```python
from build123d import *

# Parameters (mm, degrees)
SKETCH1_W           = 15
SKETCH1_H           = 4
BOSS_EXTRUDE1_DEPTH = 15
SKETCH2_W           = 15
SKETCH2_H           = 5
BOSS_EXTRUDE2_DEPTH = 15
FILLET1_R           = 1
FILLET3_R           = 5
SKETCH3_R           = 5
CUT_EXTRUDE1_DEPTH  = 3.2
SKETCH4_R           = 1.6
CUT_EXTRUDE2_DEPTH  = 26.980762229
FILLET4_R           = 5


with BuildPart() as part:
    # Sketch1 → Boss-Extrude1 (new body)
    with BuildSketch(Plane(origin=(0, 0, 0), x_dir=(1, 0, 0), z_dir=(0, 1, 0))):
        with Locations((7.5, 2)):
            Rectangle(SKETCH1_W, SKETCH1_H)
    extrude(amount=BOSS_EXTRUDE1_DEPTH)

    # Sketch2 → Boss-Extrude2 (add)
    with BuildSketch(Plane.XY):
        with Locations((7.5, 12.5)):
            Rectangle(SKETCH2_W, SKETCH2_H)
    extrude(amount=BOSS_EXTRUDE2_DEPTH)

    # Fillet1
    fillet1_edges = [part.edges().sort_by_distance(p)[0] for p in [
        (7.5, 10, 0),
    ]]
    fillet(fillet1_edges, radius=FILLET1_R)

    # Fillet3
    # the kernel refuses this fillet: 5 mm, written as the material it takes off along each edge
    with BuildSketch(Plane(origin=(5, 15, 10), x_dir=(0, -1, 0), z_dir=(-1, 0, 0))) as fillet3_piece_1_section:
        Polygon((0, 0), (FILLET3_R * 1.02, 0), (FILLET3_R * 1.02, FILLET3_R * 1.02), (0, FILLET3_R * 1.02), align=None)
    fillet3_piece_1 = extrude(amount=FILLET3_R * 1.02, mode=Mode.PRIVATE)
    fillet3_piece_1 = fillet3_piece_1 - Plane(origin=(5, 15, 10), x_dir=(0, 0.7071067811865475, -0.7071067811865475), z_dir=(-1, 0, 0)) * Sphere(FILLET3_R, mode=Mode.PRIVATE)
    add(fillet3_piece_1, mode=Mode.SUBTRACT)
    with BuildSketch(Plane(origin=(10, 15, 10), x_dir=(0, -1, 0), z_dir=(1, 0, 0))) as fillet3_piece_2_section:
        Polygon((0, 0), (FILLET3_R * 1.02, 0), (FILLET3_R * 1.02, -FILLET3_R * 1.02), (0, -FILLET3_R * 1.02), align=None)
    fillet3_piece_2 = extrude(amount=FILLET3_R * 1.02, mode=Mode.PRIVATE)
    fillet3_piece_2 = fillet3_piece_2 - Plane(origin=(10, 15, 10), x_dir=(0, 0.7071067811865475, -0.7071067811865475), z_dir=(1, 0, 0)) * Sphere(FILLET3_R, mode=Mode.PRIVATE)
    add(fillet3_piece_2, mode=Mode.SUBTRACT)
    with BuildSketch(Plane(origin=(0, 10, 1), x_dir=(0, 1, 0), z_dir=(0, 0, 1))) as fillet3_piece_3:
        with BuildLine():
            CenterArc((FILLET3_R, -FILLET3_R), FILLET3_R, 90, 90)
            Line((0, -FILLET3_R), (0, 0))
            Line((0, 0), (FILLET3_R, 0))
        make_face()
    extrude(amount=9, mode=Mode.SUBTRACT)
    with BuildSketch(Plane(origin=(15, 10, 1), x_dir=(0, 1, 0), z_dir=(0, 0, 1))) as fillet3_piece_4:
        with BuildLine():
            CenterArc((FILLET3_R, FILLET3_R), FILLET3_R, 180, 90)
            Line((0, FILLET3_R), (0, 0))
            Line((0, 0), (FILLET3_R, 0))
        make_face()
    extrude(amount=9, mode=Mode.SUBTRACT)
    with BuildSketch(Plane(origin=(10, 10, 15), x_dir=(0, 0, -1), z_dir=(-1, 0, 0))) as fillet3_piece_5:
        with BuildLine():
            CenterArc((FILLET3_R, -FILLET3_R), FILLET3_R, 90, 90)
            Line((0, -FILLET3_R), (0, 0))
            Line((0, 0), (FILLET3_R, 0))
        make_face()
    extrude(amount=5, mode=Mode.SUBTRACT)
    with BuildSketch(Plane(origin=(0, -12.5, 0), x_dir=(1, 0, 0), z_dir=(0, 1, 0))) as fillet3_piece_6:
        with BuildLine():
            CenterArc((FILLET3_R, FILLET3_R), FILLET3_R, 180, 90)
            Line((0, FILLET3_R), (0, 0))
            Line((0, 0), (FILLET3_R, 0))
        make_face()
    extrude(amount=21.5, mode=Mode.SUBTRACT)
    with BuildSketch(Plane(origin=(15, -12.5, 0), x_dir=(-1, 0, 0), z_dir=(0, 1, 0))) as fillet3_piece_7:
        with BuildLine():
            CenterArc((FILLET3_R, -FILLET3_R), FILLET3_R, 90, 90)
            Line((0, -FILLET3_R), (0, 0))
            Line((0, 0), (FILLET3_R, 0))
        make_face()
    extrude(amount=21.5, mode=Mode.SUBTRACT)
    with BuildSketch(Plane(origin=(15, 9, 1), x_dir=(0, 0, -1), z_dir=(0, -1, 0))) as fillet3_piece_8:
        with BuildLine():
            CenterArc((1 + FILLET3_R, -FILLET3_R), FILLET3_R, 90, 90)
            Line((1, -FILLET3_R), (1, 0))
            Line((1, 0), (1 + FILLET3_R, 0))
        make_face()
    revolve(axis=Axis((15, 9, 1), (1, 0, 0)), revolution_arc=90, mode=Mode.SUBTRACT)
    with BuildSketch(Plane(origin=(0, 9, 1), x_dir=(0, 0, -1), z_dir=(0, -1, 0))) as fillet3_piece_9:
        with BuildLine():
            CenterArc((1 + FILLET3_R, FILLET3_R), FILLET3_R, 180, 90)
            Line((1 + FILLET3_R, 0), (1, 0))
            Line((1, 0), (1, FILLET3_R))
        make_face()
    revolve(axis=Axis((0, 9, 1), (1, 0, 0)), revolution_arc=90, mode=Mode.SUBTRACT)

    # Sketch3 → Cut-Extrude1 (cut)
    with BuildSketch(Plane(origin=(0, 15, 0), x_dir=(1, 0, 0), z_dir=(0, 1, 0))):
        with Locations(Location((7.5, -6, 0), (0, 0, 270))):
            Circle(SKETCH3_R)
    extrude(amount=-CUT_EXTRUDE1_DEPTH, mode=Mode.SUBTRACT)

    # Sketch4 → Cut-Extrude2 (cut, through all)
    with BuildSketch(Plane.XY):
        with Locations((7.601020514, 5)):
            Circle(SKETCH4_R)
    extrude(amount=-CUT_EXTRUDE2_DEPTH, mode=Mode.SUBTRACT)

    # Fillet4
    # the kernel refuses this fillet: 5 mm, written as the material it takes off along each edge
    with BuildSketch(Plane(origin=(5, 0, -5), x_dir=(0, 0, 1), z_dir=(1, 0, 0))) as fillet4_piece_1:
        with BuildLine():
            CenterArc((5 - FILLET4_R, -FILLET4_R), FILLET4_R, 0, 90)
            Line((5 - FILLET4_R, 0), (5, 0))
            Line((5, 0), (5, -FILLET4_R))
        make_face()
    revolve(axis=Axis((5, 0, -5), (0, -1, 0)), revolution_arc=221.746220733, mode=Mode.SUBTRACT)
    with BuildSketch(Plane(origin=(10, 0, -5), x_dir=(-0.6658324541231062, 0, -0.7461012954260312), z_dir=(-0.7461012954260312, 0, 0.6658324541231062))) as fillet4_piece_2:
        with BuildLine():
            CenterArc((5 - FILLET4_R, -FILLET4_R), FILLET4_R, 0, 90)
            Line((5 - FILLET4_R, 0), (5, 0))
            Line((5, 0), (5, -FILLET4_R))
        make_face()
    revolve(axis=Axis((10, 0, -5), (0, -1, 0)), revolution_arc=221.746220733, mode=Mode.SUBTRACT)
    with BuildSketch(Plane(origin=(5, 0, 0), x_dir=(0, 1, 0), z_dir=(1, 0, 0))) as fillet4_piece_3:
        with BuildLine():
            CenterArc((FILLET4_R, -FILLET4_R), FILLET4_R, 90, 90)
            Line((0, -FILLET4_R), (0, 0))
            Line((0, 0), (FILLET4_R, 0))
        make_face()
    extrude(amount=5, mode=Mode.SUBTRACT)


solid = part.part
```
Work out the finished part from the listing and answer in its coordinate system (mm). A direction names the side the tool comes from. Give positions to 0.01 mm unless a question says otherwise; leave off trailing zeros. Order: outer loops, then holes, each group sorted by start corner. A loop starts at its lowest first (then second) coordinate and runs counter-clockwise, first axis right, second up. Notation, with made-up numbers: M -5.5,23 L 4.5,23 A11 cw 4.5,30 Z; hole C -30,37.5 d9. An arc over 180 degrees is marked long. Return JSON: item names as keys, results as strings.
1) For a pull along X with two mould halves and no side action, classify faces 5 (the flat face through (8, 11.8, 6)), 6 (the cylindrical face through (7.393, 6.586, -1.972)), 7 (the flat face through (7, 10, 5)), 8 (the flat face through (15, 14, -3)) as +X half, -X half, draft (parallel to the pull), parting line (faces both ways), or undercut.
Resolved:
{"face 5": "undercut", "face 6": "undercut", "face 7": "draft", "face 8": "+X half"}
2) Section B-B, the plane y = 3.75 is taken. Write down the section's boundary in (x, z).
Resolved:
{"outline": "M 0.26,-4 L 6.6,-4 L 6.6,-0.16 L 5,-0.16 A4.84 ccw Z; M 8.6,-4 L 14.74,-4 A4.84 ccw 10,-0.16 L 8.6,-0.16 Z"}
3) Straight lines are drawn through the part: line 1 along Y through (x, z) = (9.5, 2.25); line 2 along Y through (x, z) = (6.5, -2.25); line 3 along Z through (x, y) = (6.5, 9). For each, find the intervals that lie inside material, in ascending order. Write a range as [from, to].
Resolved:
{"line 1": "[10, 11.8]", "line 2": "[0.82, 3.84], [6.16, 15]", "line 3": "[-4, 0]"}
4) Each of these flat-tipped pins is pushed along its axis until it touches: pin 1 (1 mm diameter, centred on y = 9, z = -0.5, fed in from +X); pin 2 (1 mm diameter, centred on x = 9, z = 3.5, fed in from -Y); pin 3 (3 mm diameter, centred on x = 6.5, y = 6, fed in from +Z). Where does it stop, or does it pass through?
Resolved:
{"pin 1": "x = 13", "pin 2": "y = 10", "pin 3": "z = 0"}
5) Section C-C, the plane x = 6.25 is taken. Write down the section's boundary in (y, z).
Resolved:
{"outline": "M 0.1,-4 L 4.14,-4 L 4.14,-0.07 A5 ccw Z; M 5.86,-4 L 15,-4 L 15,1.16 L 11.8,1.16 L 11.8,10.84 L 15,10.84 L 15,15 A5 ccw 10,10 L 10,1 A1 cw 9,0 L 5.86,0 Z"}
6) Section D-D, the plane x = 1.25 is taken. Write down the section's boundary in (y, z), plus the area to 3 significant figures.
Resolved:
{"outline": "M 1.85,-4 L 15,-4 L 15,13.31 A3.31 ccw 11.69,10 L 11.69,1 A2.69 cw 9,-1.69 L 5,-1.69 A3.31 ccw Z", "area": "77.2 mm^2"}
7) Section A-A, the plane z = 6 is taken. Write down the section's boundary in (x, y).
Resolved:
{"outline": "M 0,15 A5 ccw 5,10 L 10,10 A5 ccw 15,15 L 12.5,15 L 12.5,11.8 L 2.5,11.8 L 2.5,15 Z"}
8) A tool of negligible diameter and unlimited length cuts with its end or side. For faces 1 (the cylindrical face through (13, 11, 5)), 2 (the flat face through (7, 7, 0)), 3 (the cylindrical face through (2, 7, -1)), 4 (the cylindrical face through (12.457, 13.422, 5.349)), from which of +Z, -Z, +X, -X, +Y, -Y can it reach the whole face along a straight path? Write none if from no direction.
Resolved:
{"face 1": "+Z, +X, -Y", "face 2": "+Z, +X, -X, -Y", "face 3": "+Z, -X, -Y", "face 4": "+Y"}
